```python
from build123d import *

# Parameters (mm, degrees)
F2_R      = 1.55
F2_R_2    = 12
F4_DEPTH  = 4
F3_R      = 3
F5_DEPTH  = 5
F6_DEPTH  = 16
F2_W      = 50.3
F2_H      = 3.7
F8_DEPTH  = 29
F10_DEPTH = 25


with BuildPart() as f4:
    # F2 (on Front) → F4 (new body)
    with BuildSketch(Plane.XZ):
        Polygon((29.15, -21.45), (29.15, 21.45), (-21.15, 21.45), (-21.15, 21.15), (-21.15, -21.45), (21.45, -21.45), align=None)
        with Locations((-15.5, -15.5)):
            Circle(F2_R, mode=Mode.SUBTRACT)
        Circle(F2_R_2, mode=Mode.SUBTRACT)
        with Locations((15.5, -15.5)):
            Circle(F2_R, mode=Mode.SUBTRACT)
        with Locations((-15.5, 15.5)):
            Circle(F2_R, mode=Mode.SUBTRACT)
        with Locations((15.5, 15.5)):
            Circle(F2_R, mode=Mode.SUBTRACT)
    extrude(amount=-F4_DEPTH)



with BuildPart() as f5:
    # F3 (on Right) → F5 (new body)
    with BuildSketch(Plane.YZ):
        Polygon((29, 66.85), (0, 66.85), (-57, 66.85), (-57, 40.85), (-57, 4.85), (-46, 4.85), (-46, 32.5), (0, 32.5), (0, 0), (0, -1.5), (-46, -1.5), (-46, -20.15), (-28, -20.15), (0, -20.15), (0, -40.15), (29, -40.15), align=None)
        with Locations((6.5, -33.65)):
            Circle(F3_R, mode=Mode.SUBTRACT)
        with Locations((22.5, -33.65)):
            Circle(F3_R, mode=Mode.SUBTRACT)
        with Locations((-50.5, 60.35)):
            Circle(F3_R, mode=Mode.SUBTRACT)
        with Locations((-34.5, 60.35)):
            Circle(F3_R, mode=Mode.SUBTRACT)
        with Locations((6.5, 60.35)):
            Circle(F3_R, mode=Mode.SUBTRACT)
        with Locations((22.5, 60.35)):
            Circle(F3_R, mode=Mode.SUBTRACT)
        Polygon((-46, 4.85), (-57, 4.85), (-57, -20.15), (-46, -20.15), (-46, -1.5), align=None)
        Polygon((-46, -20.15), (-57, -20.15), (-57, -40.15), (-28, -40.15), (-28, -20.15), align=None)
        with Locations((-50.5, -33.65)):
            Circle(F3_R, mode=Mode.SUBTRACT)
        with Locations((-34.5, -33.65)):
            Circle(F3_R, mode=Mode.SUBTRACT)
    extrude(amount=-F5_DEPTH)

    # F3 (on Right) → F6 (join)
    with BuildSketch(Plane.YZ):
        Polygon((-46, 4.85), (-57, 4.85), (-57, -20.15), (-46, -20.15), (-46, -1.5), align=None)
    extrude(amount=-F6_DEPTH)


with BuildPart() as f5_1:
    # F7: moved
    add(f5.part.moved(Location((33.15, 0, 0))))


with BuildPart() as f4_1:
    add(f4.part)

    add(f5_1.part)  # F8 merges F5
    # F2 (on Front) → F8 (join, through all)
    with BuildSketch(Plane.XZ):
        Polygon((-21.15, -25.15), (29.15, -25.15), (29.15, -21.45), (21.45, -21.45), (-21.15, -21.45), align=None)
        with Locations((4, 23.3)):
            Rectangle(F2_W, F2_H)
    extrude(amount=-F8_DEPTH)

    # F9 (on face) → F10 (cut, through all)
    with BuildSketch(Plane(origin=(0, 0, -20.15), x_dir=(1, 0, 0), z_dir=(0, 0, -1))):
        with BuildLine():
            Line((9.1694937954, 50), (18.9419007565, 50))
            ThreePointArc((18.9419007565, 50), (26.65, 51.5), (18.9419007565, 53))
            Line((18.9419007565, 53), (9.1694937954, 53))
            Line((9.1694937954, 53), (9.1694937954, 50))
        make_face()
    extrude(amount=-F10_DEPTH, mode=Mode.SUBTRACT)


solid = f4_1.part
```
Could you check a few things on this model? Use its own coordinates, in mm. A direction names the side the tool comes from. Coordinates: 2 decimals unless noted, no trailing zeros. Loops run counter-clockwise (first coordinate to the right, second up) from the corner with the lowest first, then second, coordinate; pieces in that order, holes last. Notation, with made-up numbers: M 6,76.5 L 34,76.5 A26 cw 34,100.5 Z; hole C 81.25,-1 d6. An arc over 180 degrees is marked long. Put each result on its own line as item: value. Start each with the question number.
(1) Suppose I cut it at B-B on y = 22.5. Please give me the cut outline in (x, z), then the cut area to 3 significant figures.
(2) Will these pins go through, and if not, where does the flat tip stop? P1, Ø12, axis at x = 26, z = 11, coming from the -Y side; P2, Ø2.5, axis at x = 15.5, z = -15.5, coming from the +Y side; P3, Ø1.2, axis at y = -54, z = -11.5, coming from the -X side; P4, Ø1, axis at x = -8, z = 23, coming from the -Y side.
(3) For faces 4 (the face through (31, -23, -1.5)), 5 (the face through (3, 14, -25.15)), 6 (the face through (4, 16, -21.45)), which set-ups out of +Z, -Z, +X, -X, +Y, -Y let a thin tool reach every point of the face, with its end or its side?
(4) Suppose I cut it at C-C on z = 60.35. Please give me the cut outline in (x, y), then the cut area to 3 significant figures.
(5) Suppose I cut it at A-A on z = -33.65. Please give me the cut outline in (x, y).
(6) Suppose I cut it at D-D on x = 15.5. Please give me the cut outline in (y, z).
(7) Thinking about a two-plate mould opening in X: for faces 1 (the face through (26.647, -51.346, -7.825)), 2 (the face through (30.68, 21.85, -36.58)), 3 (the face through (-21.15, 3.7, 0.1)), which applies, pulls with the +X half, pulls with the -X half, needs draft (parallel to the pull), parting line crosses it, or undercut?
(8) I need wall thicknesses on line 1 (X direction, y = 2, z = 15); line 2 (Z direction, x = 7, y = 13); line 3 (Z direction, x = 0, y = 1.65). Which ranges of each line are inside material? Lowest first, please. Write a range as from..to.
Solutions:
1. outline: M -21.15,-25.15 L 28.15,-25.15 L 28.15,-30.65 L 33.15,-30.65 L 33.15,57.35 L 28.15,57.35 L 28.15,25.15 L -21.15,25.15 L -21.15,21.45 L 28.15,21.45 L 28.15,-21.45 L -21.15,-21.45 Z; M 28.15,-40.15 L 33.15,-40.15 L 33.15,-36.65 L 28.15,-36.65 Z; M 28.15,63.35 L 33.15,63.35 L 33.15,66.85 L 28.15,66.85 Z
1. area: 840 mm2
2. P1: stops at y = -57
2. P2: passes through
2. P3: stops at x = 17.15
2. P4: stops at y = 0
3. face 4: +X, -X
3. face 5: -Z, -X, +Y, -Y
3. face 6: -X, +Y
4. outline: M 28.15,-57 L 33.15,-57 L 33.15,-53.5 L 28.15,-53.5 Z; M 28.15,-47.5 L 33.15,-47.5 L 33.15,-37.5 L 28.15,-37.5 Z; M 28.15,-31.5 L 33.15,-31.5 L 33.15,3.5 L 28.15,3.5 Z; M 28.15,9.5 L 33.15,9.5 L 33.15,19.5 L 28.15,19.5 Z; M 28.15,25.5 L 33.15,25.5 L 33.15,29 L 28.15,29 Z
4. area: 310 mm2
5. outline: M 28.15,-57 L 33.15,-57 L 33.15,-53.5 L 28.15,-53.5 Z; M 28.15,-47.5 L 33.15,-47.5 L 33.15,-37.5 L 28.15,-37.5 Z; M 28.15,-31.5 L 33.15,-31.5 L 33.15,-28 L 28.15,-28 Z; M 28.15,0 L 33.15,0 L 33.15,3.5 L 28.15,3.5 Z; M 28.15,9.5 L 33.15,9.5 L 33.15,19.5 L 28.15,19.5 Z; M 28.15,25.5 L 33.15,25.5 L 33.15,29 L 28.15,29 Z
6. outline: M 0,-25.15 L 29,-25.15 L 29,-21.45 L 4,-21.45 L 4,-17.05 L 0,-17.05 Z; M 0,-13.95 L 4,-13.95 L 4,13.95 L 0,13.95 Z; M 0,17.05 L 4,17.05 L 4,21.45 L 29,21.45 L 29,25.15 L 0,25.15 Z
7. face 1: undercut
7. face 2: needs draft
7. face 3: pulls with the -X half
8. line 1: x = -21.15..-16.97, -14.03..14.03, 16.97..33.15
8. line 2: z = -25.15..-21.45, 21.45..25.15
8. line 3: z = -25.15..-12, 12..25.15
